The listing builds one solid part. Answer for the finished solid, in the listing's coordinates (mm). A direction names the side the tool comes from. Round coordinates to 2 decimals unless told otherwise and drop trailing zeros. Loops run counter-clockwise (first coordinate to the right, second up) from the corner with the lowest first, then second, coordinate; pieces in that order, holes last. Notation, with made-up numbers: (25, -16.75) -> (52, -16.75) arc R21 cw to (52, 20.25) -> close; hole circle Ø5 at (13.25, 13.25). An arc over 180 degrees is marked (long way). Write each question's results on one line, items separated by ' | '. Start each with the question number.
(1) The part is cut by section A-A (x = -10). Determine the outline of the cut face in (y, z).
(2) Straight lines are drawn through the part: probe 1 along X at (y, z) = (2.2, 6.3); probe 2 along Z at (x, y) = (5.5, 3.5); probe 3 along Z at (x, y) = (-10, 1.55). For each, find the intervals that lie inside material, in ascending order.
(3) Determine the mould class of faces 1 (the face through (10.03, 2.54, 7.25)), 2 (the face through (9.97, 2.54, -7.25)), 3 (the face through (25, 2, 0)), 4 (the face through (0, 2, -10)) for opening direction Z: released by +Z, released by -Z, zero draft, split by the parting line, or undercut.
(4) For faces 5 (the face through (0, 0, 0)), 6 (the face through (-14, 4, 5.35)), 7 (the face through (21, 4, 4)), 8 (the face through (-10, 1, -5.35)), determine the directions among +Z, -Z, +X, -X, +Y, -Y from which every point of the face is accessible in a straight line to the end or side of a thin tool.
(5) The part is cut by section C-C (y = 1.05). Determine the outline of the cut face in (x, z), plus the area to 3 significant figures.
(6) The part is cut by section B-B (z = -6.3). Determine the outline of the cut face in (x, y), plus the area to 3 significant figures.
(7) A flat-ended cylindrical pin translates along its axis: pin 1 (1 mm diameter, centred on x = -6.5, z = -3, fed in from +Y). Find the tip coordinate at first contact, or state that the pin passes through.
```python
from build123d import *

# Parameters (mm, degrees)
EXTRUDE_1_DEPTH     = 5
CUT_EXTRUDE_1_DEPTH = 2.8
CUT_EXTRUDE_2_DEPTH = 5


with BuildPart() as part:
    # 草圖1 → 填料-伸長1 (new body)
    with BuildSketch(Plane(origin=(0, 0, 0), x_dir=(1, 0, 0), z_dir=(0, 1, 0))):
        with BuildLine():
            Line((-23, -10), (23, -10))
            ThreePointArc((23, -10), (24.414213562, -9.414213562), (25, -8))
            Line((25, -8), (25, 8))
            ThreePointArc((25, 8), (24.414213562, 9.414213562), (23, 10))
            Line((23, 10), (-23, 10))
            ThreePointArc((-23, 10), (-24.414213562, 9.414213562), (-25, 8))
            Line((-25, 8), (-25, -8))
            ThreePointArc((-25, -8), (-24.414213562, -9.414213562), (-23, -10))
        make_face()
    extrude(amount=EXTRUDE_1_DEPTH)

    # 草圖2 → 除料-伸長1 (cut)
    with BuildSketch(Plane(origin=(0, 5, 0), x_dir=(1, 0, 0), z_dir=(0, 1, 0))):
        Polygon((-17.35, -5.35), (17.35, -5.35), (17.35, -4), (25, -4), (25, 4), (17.35, 4), (17.35, 5.35), (-17.35, 5.35), align=None)
    extrude(amount=-CUT_EXTRUDE_1_DEPTH, mode=Mode.SUBTRACT)

    # 草圖3 → 除料-伸長2 (cut)
    with BuildSketch(Plane(origin=(0, 5, 0), x_dir=(1, 0, 0), z_dir=(0, 1, 0))):
        with BuildLine():
            Line((-10.6, 5.563454007), (-10.6, 5.35))
            Line((-10.6, 5.35), (-9.4, 5.35))
            Line((-9.4, 5.35), (-9.4, 5.563454007))
            ThreePointArc((-9.4, 5.563454007), (-10, 7.25), (-10.6, 5.563454007))
        make_face()
        with BuildLine():
            Line((-10.6, -5.35), (-9.4, -5.35))
            Line((-9.4, -5.35), (-9.4, -5.563454007))
            ThreePointArc((-9.4, -5.563454007), (-10, -7.25), (-10.6, -5.563454007))
            Line((-10.6, -5.563454007), (-10.6, -5.35))
        make_face()
        with BuildLine():
            Line((10.6, 5.563454007), (10.6, 5.35))
            Line((10.6, 5.35), (9.4, 5.35))
            Line((9.4, 5.35), (9.4, 5.563454007))
            ThreePointArc((9.4, 5.563454007), (10, 7.25), (10.6, 5.563454007))
        make_face()
        with BuildLine():
            Line((9.4, -5.563454007), (9.4, -5.35))
            Line((9.4, -5.35), (10.6, -5.35))
            Line((10.6, -5.35), (10.6, -5.563454007))
            ThreePointArc((10.6, -5.563454007), (10, -7.25), (9.4, -5.563454007))
        make_face()
    extrude(amount=-CUT_EXTRUDE_2_DEPTH, mode=Mode.SUBTRACT)


solid = part.part
```
Checked values:
1) outline: (0, -10) -> (5, -10) -> (5, -7.25) -> (0, -7.25) -> close; (0, -5.35) -> (2.2, -5.35) -> (2.2, 5.35) -> (0, 5.35) -> close; (0, 7.25) -> (5, 7.25) -> (5, 10) -> (0, 10) -> close
2) probe 1: x = -25 to -10.95, -9.05 to 9.05, 10.95 to 25 | probe 2: z = -10 to -5.35, 5.35 to 10 | probe 3: z = -10 to -7.25, -5.35 to 5.35, 7.25 to 10
3) face 1: undercut | face 2: undercut | face 3: zero draft | face 4: released by -Z
4) face 5: +Z, -Z, +X, -X, -Y | face 6: +Y | face 7: +X, +Y | face 8: +Y, -Y
5) outline: (-25, -8) arc R2 ccw to (-23, -10) -> (23, -10) arc R2 ccw to (25, -8) -> (25, 8) arc R2 ccw to (23, 10) -> (-23, 10) arc R2 ccw to (-25, 8) -> close; hole (-10.6, -5.56) arc R0.95 ccw (long way) to (-9.4, -5.56) -> (-9.4, -5.35) -> (-10.6, -5.35) -> close; hole (-10.6, 5.35) -> (-9.4, 5.35) -> (-9.4, 5.56) arc R0.95 ccw (long way) to (-10.6, 5.56) -> close; hole (9.4, -5.56) arc R0.95 ccw (long way) to (10.6, -5.56) -> (10.6, -5.35) -> (9.4, -5.35) -> close; hole (9.4, 5.35) -> (10.6, 5.35) -> (10.6, 5.56) arc R0.95 ccw (long way) to (9.4, 5.56) -> close | area: 985 mm2
6) outline: (-25, 0) -> (-10.95, 0) -> (-10.95, 5) -> (-25, 5) -> close; (-9.05, 0) -> (9.05, 0) -> (9.05, 5) -> (-9.05, 5) -> close; (10.95, 0) -> (25, 0) -> (25, 5) -> (10.95, 5) -> close | area: 231 mm2
7) pin 1: stops at y = 2.2
